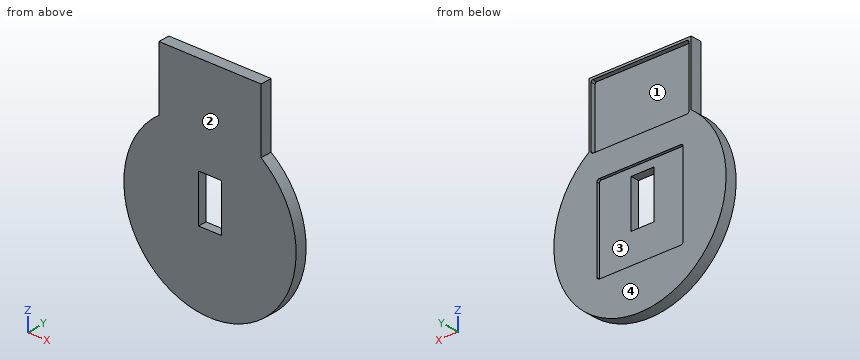
```python
from build123d import *

# Parameters (mm, degrees)
BOSS_EXTRUDE2_DEPTH = 10
CUT_EXTRUDE2_START  = 10
SKETCH3_W           = 75
SKETCH3_H           = 75
CUT_EXTRUDE2_DEPTH  = 2.5
FILLET2_R           = 2
CUT_EXTRUDE3_START  = 10
SKETCH5_W           = 85
SKETCH5_H           = 55
CUT_EXTRUDE3_DEPTH  = 4
FILLET3_R           = 1.5
CUT_EXTRUDE4_START  = 7.5
SKETCH6_W           = 20
SKETCH6_H           = 41
CUT_EXTRUDE4_DEPTH  = 45


with BuildPart() as part:
    # Sketch2 → Boss-Extrude2 (new body)
    with BuildSketch(Plane(origin=(0, 0, 0), x_dir=(1, 0, 0), z_dir=(0, 1, 0))):
        with BuildLine():
            Line((-44.5, -60.371764924), (-44.5, -115.371764924))
            Line((-44.5, -115.371764924), (44.5, -115.371764924))
            Line((44.5, -115.371764924), (44.5, -60.371764924))
            ThreePointArc((44.5, -60.371764924), (0, 75), (-44.5, -60.371764924))
        make_face()
    extrude(amount=BOSS_EXTRUDE2_DEPTH)

    # Sketch3 → Cut-Extrude2 (cut)
    with BuildSketch(Plane(origin=(0, 0, 0), x_dir=(1, 0, 0), z_dir=(0, 1, 0)).offset(CUT_EXTRUDE2_START)):
        Rectangle(SKETCH3_W, SKETCH3_H)
    extrude(amount=-CUT_EXTRUDE2_DEPTH, mode=Mode.SUBTRACT)

    # Fillet2
    fillet2_edges = [part.edges().sort_by_distance(p)[0] for p in [
        (37.5, 8.75, -37.5),
        (37.5, 8.75, 37.5),
        (-37.5, 8.75, 37.5),
        (-37.5, 8.75, -37.5),
    ]]
    fillet(fillet2_edges, radius=FILLET2_R)

    # Sketch5 → Cut-Extrude3 (cut)
    with BuildSketch(Plane(origin=(0, 0, 0), x_dir=(1, 0, 0), z_dir=(0, 1, 0)).offset(CUT_EXTRUDE3_START)):
        with Locations((0, -85.871764924)):
            Rectangle(SKETCH5_W, SKETCH5_H)
    extrude(amount=-CUT_EXTRUDE3_DEPTH, mode=Mode.SUBTRACT)

    # Fillet3
    fillet3_edges = [part.edges().sort_by_distance(p)[0] for p in [
        (42.5, 8, 113.371764924),
        (-42.5, 8, 113.371764924),
        (-42.5, 8, 58.371764924),
        (42.5, 8, 58.371764924),
    ]]
    fillet(fillet3_edges, radius=FILLET3_R)

    # Sketch6 → Cut-Extrude4 (cut)
    with BuildSketch(Plane(origin=(0, 0, 0), x_dir=(1, 0, 0), z_dir=(0, 1, 0)).offset(CUT_EXTRUDE4_START)):
        with Locations((0, -10.5)):
            Rectangle(SKETCH6_W, SKETCH6_H)
    extrude(amount=-CUT_EXTRUDE4_DEPTH, mode=Mode.SUBTRACT)


solid = part.part
```
Verification items for the finished model (mm, model axes). Face numbers are marked on the shaded views. A direction names the side the tool comes from. Coordinates: 2 decimals unless noted, no trailing zeros. Write each loop counter-clockwise with the first axis right and the second up, starting at its lowest first coordinate (ties: lowest second). Pieces come first, ordered by that corner, then holes. Notation, with made-up numbers: M 61,-27 L 66,-27 A28 cw 66,6 Z; hole C -31,29.5 d10. An arc over 180 degrees is marked long. Answer as a JSON object with one key per item and string values. Group by question number.
(1) Cross-section at D-D, the plane z = -29. Record the cut outline in (x, y), and give its area (3 significant figures).
(2) Material ranges on line 1 (Y direction, x = 21.5, z = 82.5); line 2 (Z direction, x = -38.5, y = 6.5); line 3 (X direction, y = 7, z = 100), recorded low to high.
(3) Release check for a two-part mould opening along Z. For the marked faces 3 and 4 record: +Z half, -Z half, draft (parallel to the pull), parting line (faces both ways), or undercut.
(4) Cross-section at B-B, the plane z = 0. Record the cut outline in (x, y), and give its area (3 significant figures).
(5) Tool access check on the marked faces 1 and 2. Record the directions out of +Z, -Z, +X, -X, +Y, -Y that give a thin tool (end or side, any length) a straight path to the whole face; none if there is none.
(6) Cross-section at C-C, the plane y = 3. Record the cut outline in (x, z), and give its area (3 significant figures).
(7) Gauge pin test, flat ends, axial feed: pin 1 (1.2 mm diameter, centred on y = 8.5, z = -17, fed in from -X) (3 decimals); pin 2 (1.2 mm diameter, centred on y = 7, z = 92, fed in from +X); pin 3 (6 mm diameter, centred on y = 2.5, z = 8.5, fed in from +X); pin 4 (4 mm diameter, centred on x = -1.5, y = 4, fed in from -Z). Record the tip position at first contact, or that the pin passes through.
(8) Cross-section at A-A, the plane x = 0. Record the cut outline in (y, z).
Reply:
{
 "1": {"outline": "M -69.17,0 L 69.17,0 L 69.17,10 L 37.5,10 L 37.5,7.5 L -37.5,7.5 L -37.5,10 L -69.17,10 Z", "area": "1,200 mm²"},
 "2": {"line 1": "0 to 6", "line 2": "-64.36 to 58.37, 113.37 to 115.37", "line 3": "-44.5 to -42.5, 42.5 to 44.5"},
 "3": {"face 3": "undercut", "face 4": "draft"},
 "4": {"outline": "M -75,0 L -10,0 L -10,7.5 L -37.5,7.5 L -37.5,10 L -75,10 Z; M 10,0 L 75,0 L 75,10 L 37.5,10 L 37.5,7.5 L 10,7.5 Z", "area": "1,160 mm²"},
 "5": {"face 1": "+Y", "face 2": "+Z, -Z, +X, -X, -Y"},
 "6": {"outline": "M -44.5,60.37 A75 ccw long 44.5,60.37 L 44.5,115.37 L -44.5,115.37 Z; hole M -10,-10 L 10,-10 L 10,31 L -10,31 Z", "area": "20,900 mm²"},
 "7": {"pin 1": "x = -73.185", "pin 2": "x = 44.5", "pin 3": "x = 74.8", "pin 4": "z = -75"},
 "8": {"outline": "M 0,-75 L 10,-75 L 10,-37.5 L 7.5,-37.5 L 7.5,-10 L 0,-10 Z; M 0,31 L 7.5,31 L 7.5,37.5 L 10,37.5 L 10,58.37 L 6,58.37 L 6,113.37 L 10,113.37 L 10,115.37 L 0,115.37 Z"}
}
